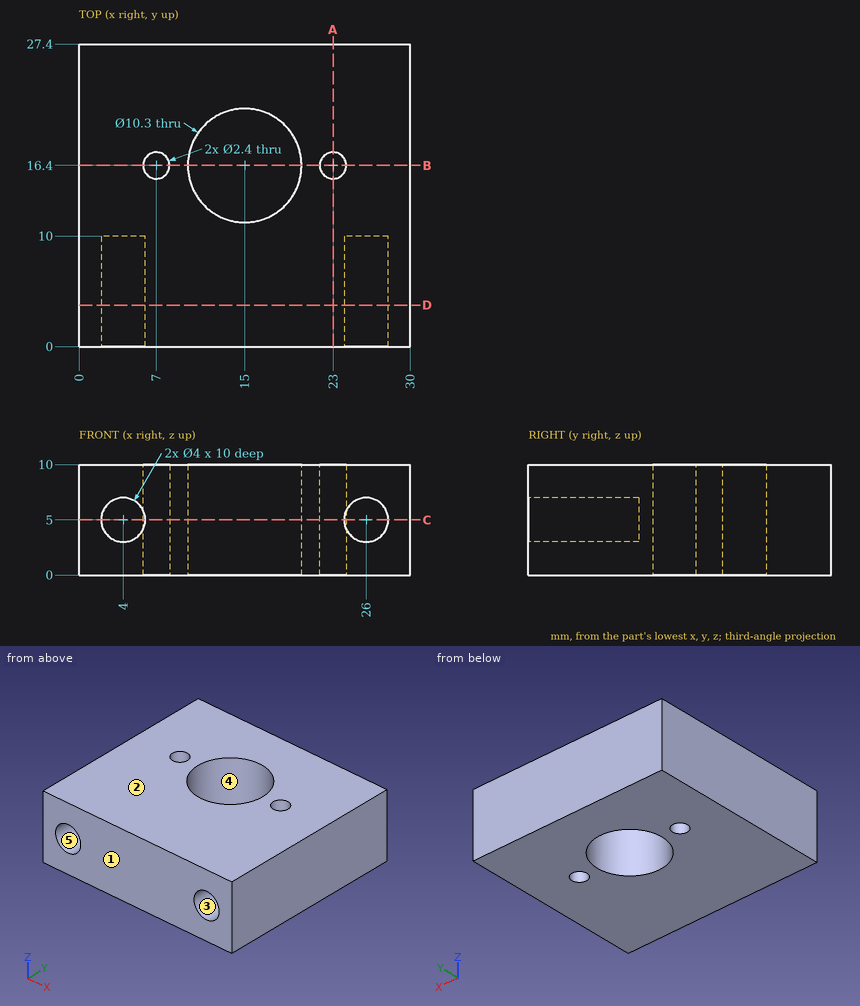
Geometry check sheet. Reference: drawing and pictorial views, mm from the part's lowest x, y, z. A direction names the side the tool comes from. Give positions to 0.01 mm unless a question says otherwise; leave off trailing zeros. Write each loop counter-clockwise with the first axis right and the second up, starting at its lowest first coordinate (ties: lowest second). Pieces come first, ordered by that corner, then holes. Notation, with made-up numbers: (10, -11.75) -> (41, -11.75) arc R33 cw to (41, 16.25) -> close; hole circle Ø7 at (33, 30). An arc over 180 degrees is marked (long way). One line per item, written item: value. Start each with the question number.
Item 1: Section check D-D on y = 3.75. Record the cut outline in (x, z), then the cut area to 3 significant figures.
Item 2: Section check C-C on z = 5. Record the cut outline in (x, y), then the cut area to 3 significant figures.
Item 3: Section check B-B on y = 16.4. Record the cut outline in (x, z), then the cut area to 3 significant figures.
Item 4: Material ranges on probe 1 along Y at (x, z) = (15, 7); probe 2 along X at (y, z) = (7.25, 4); probe 3 along Y at (x, z) = (7, 4.75), recorded low to high. Write a range as from..to.
Item 5: Section check A-A on x = 23. Record the cut outline in (y, z).
Item 6: Tool access check on the marked faces 4 and 5. Record the directions out of +Z, -Z, +X, -X, +Y, -Y that give a thin tool (end or side, any length) a straight path to the whole face; none if there is none.
Item 7: Draft check along Z on the marked faces 1, 2 and 3. Enter one of: +Z half, -Z half, draft (parallel to the pull), parting line (faces both ways), or undercut.
Item 8: Gauge pin test, flat ends, axial feed: pin 1 (1.2 mm diameter, centred on x = 26, z = 4, fed in from -Y); pin 2 (1.5 mm diameter, centred on x = 20, z = 4, fed in from -Y). Record the tip position at first contact, or that the pin passes through.
Results list:
1. outline: (0, 0) -> (30, 0) -> (30, 10) -> (0, 10) -> close; hole circle Ø4 at (4, 5); hole circle Ø4 at (26, 5)
1. area: 275 mm²
2. outline: (0, 0) -> (2, 0) -> (2, 10) -> (6, 10) -> (6, 0) -> (24, 0) -> (24, 10) -> (28, 10) -> (28, 0) -> (30, 0) -> (30, 27.4) -> (0, 27.4) -> close; hole circle Ø2.4 at (7, 16.4); hole circle Ø10.3 at (15, 16.4); hole circle Ø2.4 at (23, 16.4)
2. area: 650 mm²
3. outline: (0, 0) -> (5.8, 0) -> (5.8, 10) -> (0, 10) -> close; (8.2, 0) -> (9.85, 0) -> (9.85, 10) -> (8.2, 10) -> close; (20.15, 0) -> (21.8, 0) -> (21.8, 10) -> (20.15, 10) -> close; (24.2, 0) -> (30, 0) -> (30, 10) -> (24.2, 10) -> close
3. area: 149 mm²
4. probe 1: 0..11.25, 21.55..27.4
4. probe 2: 0..2.27, 5.73..24.27, 27.73..30
4. probe 3: 0..15.2, 17.6..27.4
5. outline: (0, 0) -> (15.2, 0) -> (15.2, 10) -> (0, 10) -> close; (17.6, 0) -> (27.4, 0) -> (27.4, 10) -> (17.6, 10) -> close
6. face 4: +Z, -Z
6. face 5: -Y
7. face 1: draft
7. face 2: +Z half
7. face 3: undercut
8. pin 1: y = 10
8. pin 2: y = 0
